The drawing under review shows one solid part. Ordinate dimensions are in mm from its lowest x, y, z. A direction names the side the tool comes from. Round coordinates to 2 decimals unless told otherwise and drop trailing zeros. Write each loop counter-clockwise with the first axis right and the second up, starting at its lowest first coordinate (ties: lowest second). Pieces come first, ordered by that corner, then holes. Notation, with made-up numbers: (-37.5, 72) -> (-23.5, 72) arc R21 cw to (-23.5, 111) -> close; hole circle Ø2 at (17.25, 75.25). An arc over 180 degrees is marked (long way). Use CSV: the item, a comma, the result in double quotes. Start each with the question number.
1) Take a section at B-B, the plane z = 21.25. Give the boundary of the cut face in (x, y).
2) For pin 1 Ø5.5 at (y, z) = (3, 23.5) entering from -X; pin 2 Ø1 at (x, z) = (13, 33) entering from -Y; pin 3 Ø6 at (y, z) = (5.5, 11.5) entering from +X, all flat-tipped, find the tip position at first contact; note any pin that passes through.
3) Machinability: for the marked faces 1, 2 and 3, which of the approach directions +Z, -Z, +X, -X, +Y, -Y give a long, thin tool a straight path to every point of the face, cutting with its end or side? Answer none if there is none.
4) Wall thickness on probe 1 along Z at (x, y) = (32, 7.75); probe 2 along Z at (x, y) = (56, 9.15); probe 3 along X at (y, z) = (8.6, 46.5) (1 decimal): over which ranges is each line inside the solid? List them lowest first. Write a range as [from, to].
5) Take a section at C-C, the plane y = 6. Give the boundary of the cut face in (x, z).
6) Take a section at A-A, the plane x = 56. Give the boundary of the cut face in (y, z), then the cut area to 3 significant figures.
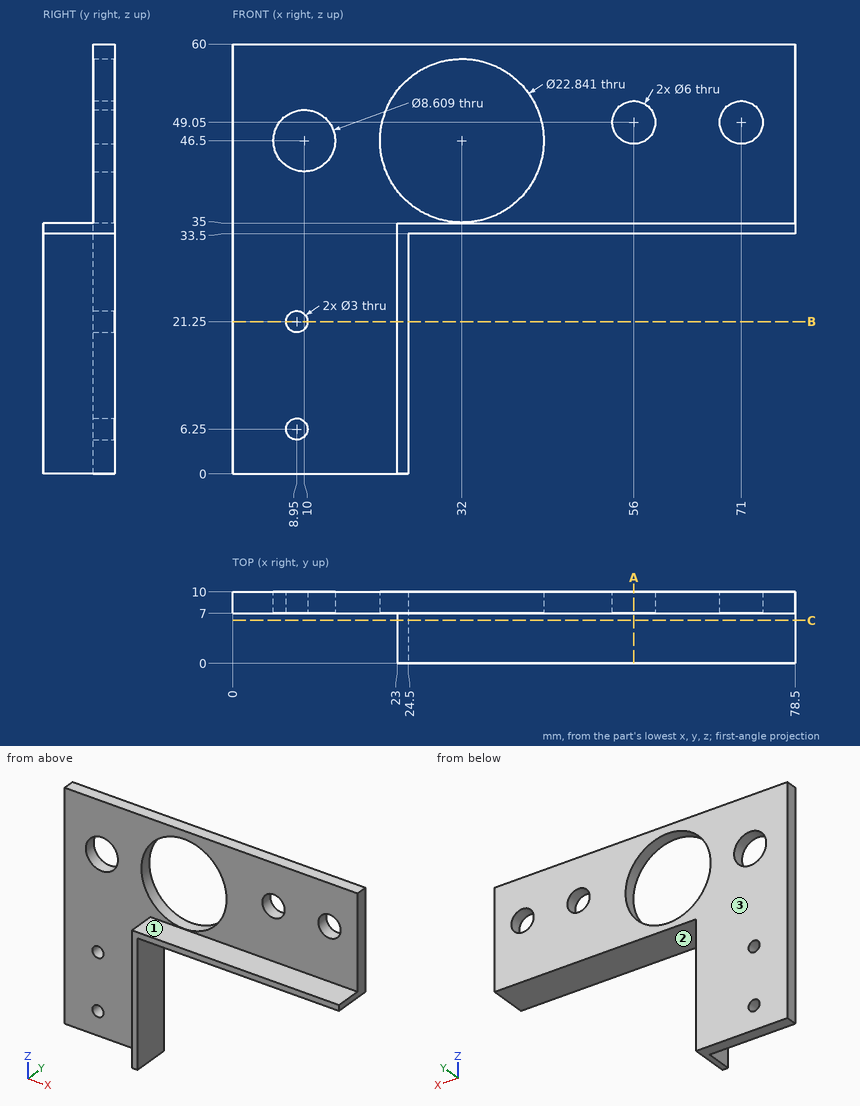
Values found:
1,outline,"(0, 7) -> (7.45, 7) -> (7.45, 10) -> (0, 10) -> close; (10.45, 7) -> (23, 7) -> (23, 0) -> (24.5, 0) -> (24.5, 10) -> (10.45, 10) -> close"
2,pin 1,"x = 23"
2,pin 2,"y = 7"
2,pin 3,"x = 24.5"
3,face 1,"+Z, +X, -X, -Y"
3,face 2,"-Z, +X, +Y, -Y"
3,face 3,"+Z, -Z, +X, -X, +Y"
4,probe 1,"[33.5, 35.08], [57.92, 60]"
4,probe 2,"[33.5, 46.05], [52.05, 60]"
4,probe 3,"[0, 5.7], [14.3, 20.6], [43.4, 54.4], [57.6, 69.4], [72.6, 78.5]"
5,outline,"(23, 0) -> (24.5, 0) -> (24.5, 33.5) -> (78.5, 33.5) -> (78.5, 35) -> (23, 35) -> close"
6,outline,"(0, 33.5) -> (10, 33.5) -> (10, 46.05) -> (7, 46.05) -> (7, 35) -> (0, 35) -> close; (7, 52.05) -> (10, 52.05) -> (10, 60) -> (7, 60) -> close"
6,area,"72.0 mm²"
